Part model, mm, in its own coordinate system. Face numbers are marked on the shaded views. A direction names the side the tool comes from. Round coordinates to 2 decimals unless told otherwise and drop trailing zeros. Write each loop counter-clockwise with the first axis right and the second up, starting at its lowest first coordinate (ties: lowest second). Pieces come first, ordered by that corner, then holes.
1) Saw through at D-D on y = 2.5. Write the cut outline in (x, z), and give its area (3 significant figures).
2) Which spindle directions (+Z, -Z, +X, -X, +Y, -Y) get a long thin tool onto all of the face, cutting with end or side? Do the marked faces 1, 2 and 3. Say none if no direction does.
3) Saw through at A-A on x = -46. Write the cut outline in (y, z), and give its area (3 significant figures).
4) Saw through at C-C on z = -14.5. Write the cut outline in (x, y).
5) Saw through at B-B on z = -27.5. Write the cut outline in (x, y).
6) Drill centre lines: L1, parallel to X at y = 13, z = -27; L2, parallel to Z at x = -37, y = 9; L3, parallel to Z at x = -35, y = 2.5. Where is each one in solid material? Low to high.
7) Flat gauge pins, fed straight in: pin 1 (8 mm diameter, centred on x = -40.5, z = -23, fed in from -Y); pin 2 (0.6 mm diameter, centred on y = -8.5, z = -6.5, fed in from -X); pin 3 (2 mm diameter, centred on x = -63.5, y = 15, fed in from +Z). Where does each tip first touch, or does it go through?
Autodesk Inventor part; units mm, degrees
ref_plane "YZ Plane" through (0, 0, 0) normal (1, 0, 0) x (0, 1, 0)
ref_plane "XZ Plane" through (0, 0, 0) normal (0, 1, 0) x (-1, 0, 0)
ref_plane "XY Plane" through (0, 0, 0) normal (0, 0, 1) x (1, 0, 0)
ref_plane "Work Plane2" through (-65.3804, 18.9113, -35.9508) normal (-1, 0, 0) x (0, -0.7071, -0.7071)
ref_plane "Work Plane3" through (-52.8804, 7.2095, -21.4206) normal (0, 0.7071, 0.7071) x (-1, 0, 0)
sketch "Sketch3" plane through (-52.8804, 7.2095, -21.4206) normal (0, 0.7071, 0.7071) x (-1, 0, 0)
  circle A0 centre (16, 5.6569) radius 1.4 construction
  circle A1 centre (-16, 5.6569) radius 1.4 construction
  line L0 (-16.9, -3.0998) -> (-16.9, -27) construction
  line L1 (14.3, 19.8) -> (12.8, 19.8) construction
  line L2 (14.3, 19.8) -> (14.3, -19.254) construction
  line L3 (12.8, 19.8) -> (12.8, -18.254) construction
  line L4 (-12.8, -18.254) -> (-12.8, 19.8) construction
  line L5 (-12.8, 19.8) -> (-14.3, 19.8) construction
  line L6 (-14.3, 19.8) -> (-14.3, -18.254) construction
  line L7 (12.8, -18.254) -> (-12.8, -18.254) construction
  line L8 (-12.5, -18.5487) -> (12.5, -18.5487) construction
  line L9 (18, -17.4431) -> (-18, -17.4431)
  line L10 (-18, -17.4431) -> (-18, 22.7569)
  line L11 (-18, 22.7569) -> (18, 22.7569)
  line L12 (18, 22.7569) -> (18, -17.4431)
  line L13 (10.8, -15.4431) -> (-12.3, -15.4431)
  line L14 (-12.3, -15.4431) -> (-12.3, 20.7569)
  line L15 (-12.3, 20.7569) -> (10.8, 20.7569)
  line L16 (10.8, 20.7569) -> (10.8, -15.4431)
  circle A2 centre (16, 5.6569) radius 1.4
  circle A3 centre (-16, 5.6569) radius 1.4
  line L17 (16, 10.5407) -> (16, 0.773) construction
  line L18 (14.6, 10.5407) -> (14.6, 0.773)
  line L19 (17.4, 0.773) -> (17.4, 10.5407)
  arc A4 (17.4, 10.5407) -> (14.6, 10.5407) centre (16, 10.5407) ccw
  arc A5 (14.6, 0.773) -> (17.4, 0.773) centre (16, 0.773) ccw
  line L20 (-16, 10.5407) -> (-16, 0.773) construction
  line L21 (-17.4, 10.5407) -> (-17.4, 0.773)
  line L22 (-14.6, 0.773) -> (-14.6, 10.5407)
  arc A6 (-14.6, 10.5407) -> (-17.4, 10.5407) centre (-16, 10.5407) ccw
  arc A7 (-17.4, 0.773) -> (-14.6, 0.773) centre (-16, 0.773) ccw
  point P0 (-52.8804, 20.2446)
  dimension "d12" = 2
  dimension "d13" = 2
  dimension "d14" = 23.1
  dimension "d15" = 17.1
  dimension "d16" = 2
  dimension "d17" = 2
  dimension "d18" = 2
  dimension "d19" = 2
extrude "Extrusion3" add sketch "Sketch3" along normal blind 1
sketch "Sketch4" plane through (-52.8804, 7.2095, -21.4206) normal (0, -0.7071, -0.7071) x (-1, 0, 0)
  line L0 (-12.3, 15.4431) -> (-12.3, -20.7569)
  line L1 (-12.3, -20.7569) -> (10.8, -20.7569)
  line L2 (10.8, -20.7569) -> (10.8, 15.4431)
  line L3 (10.8, 15.4431) -> (-12.3, 15.4431)
  line L4 (-18, 17.4431) -> (18, 17.4431)
  line L5 (18, 17.4431) -> (18, -22.7569)
  line L6 (18, -22.7569) -> (-18, -22.7569)
  line L7 (-18, -22.7569) -> (-18, 17.4431)
  line L8 (-18, 17.4431) -> (18, 17.4431)
  line L9 (-12.3, 15.4431) -> (10.8, 15.4431)
  line L10 (9.607, 17.4431) -> (-11.0714, 17.4431)
  line L11 (-11.0714, 17.4431) -> (-11.0714, 15.4431)
  line L12 (-11.0714, 15.4431) -> (9.607, 15.4431)
  line L13 (9.607, 15.4431) -> (9.607, 17.4431)
  line L14 (10.8, -20.7569) -> (-12.3, -20.7569)
  line L15 (9.607, -22.7569) -> (-11.0714, -22.7569)
  line L16 (-11.0714, -22.7569) -> (-11.0714, -20.7569)
  line L17 (-11.0714, -20.7569) -> (9.607, -20.7569)
  line L18 (9.607, -20.7569) -> (9.607, -22.7569)
  point P0 (-52.8804, -20.2446)
extrude "Extrusion4" add sketch "Sketch4" along normal blind 1 contours L11 L4 L13 L3 | L1 L18 L6 L16
sketch "Sketch5" plane through (-52.8804, 7.2095, -21.4206) normal (0, -0.7071, -0.7071) x (-1, 0, 0)
  line L0 (-18, 17.4431) -> (18, 17.4431)
  line L1 (18, -22.7569) -> (-18, -22.7569)
  line L2 (-18, -22.7569) -> (-21, -22.7569)
  line L3 (-21, -22.7569) -> (-21, 17.4431)
  line L4 (-21, 17.4431) -> (-18, 17.4431)
  line L5 (-18, 17.4431) -> (-18, -22.7569)
  line L6 (18, -22.7569) -> (21, -22.7569)
  line L7 (21, -22.7569) -> (21, 17.4431)
  line L8 (21, 17.4431) -> (18, 17.4431)
  line L9 (18, 17.4431) -> (18, -22.7569)
  point P0 (-52.8804, -20.2446)
  dimension "d24" = 3
  dimension "d25" = 3
  dimension "d28" = 40.2
extrude "Extrusion5" add sketch "Sketch5" against normal up to surface (1 mm away) contours L5 L2 L3 L4 | L8 L7 L6 L9
properties part number "20_Cube_Insert_Beamsplittercube_Dichroicmirror_Retainplate"
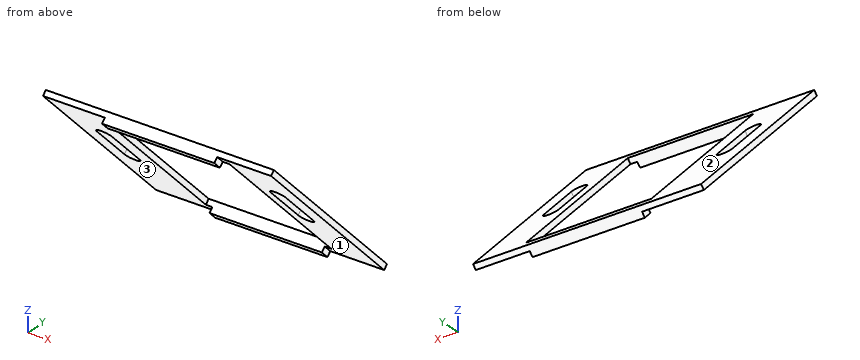
Completed:
1. outline: (-73.88, -16.71) - (-70.28, -16.71) - (-70.28, -15.3) - (-73.88, -15.3) - close; (-67.48, -16.71) - (-63.68, -16.71) - (-63.68, -15.3) - (-67.48, -15.3) - close; (-40.58, -16.71) - (-38.28, -16.71) - (-38.28, -15.3) - (-40.58, -15.3) - close; (-35.48, -16.71) - (-31.88, -16.71) - (-31.88, -15.3) - (-35.48, -15.3) - close
1. area: 18.8 mm2
2. face 1: -Z, +X, -Y
2. face 2: +Z, +X, -X, +Y
2. face 3: -Z, -X, -Y
3. outline: (-9.59, -6.04) - (-8.17, -7.45) - (-6.76, -6.04) - (-8.17, -4.62) - close; (17.42, -33.05) - (18.84, -34.46) - (20.25, -33.05) - (18.84, -31.63) - close
3. area: 8.00 mm2
4. outline: (-73.88, 0.29) - (-70.28, 0.29) - (-70.28, 1.7) - (-73.88, 1.7) - close; (-67.48, 0.29) - (-63.68, 0.29) - (-63.68, 1.7) - (-67.48, 1.7) - close; (-40.58, 0.29) - (-38.28, 0.29) - (-38.28, 1.7) - (-40.58, 1.7) - close; (-35.48, 0.29) - (-31.88, 0.29) - (-31.88, 1.7) - (-35.48, 1.7) - close
5. outline: (-73.88, 13.29) - (-63.68, 13.29) - (-63.68, 14.7) - (-73.88, 14.7) - close; (-40.58, 13.29) - (-31.88, 13.29) - (-31.88, 14.7) - (-40.58, 14.7) - close
6. L1: x = -73.88 to -63.68, -40.58 to -31.88
6. L2: z = -23.21 to -21.8
6. L3: z = -16.71 to -15.3
7. pin 1: stops at y = 4.79
7. pin 2: stops at x = -62.49
7. pin 3: stops at z = -26.81
